Geometry check sheet. Reference: the model listing, model coordinates, mm. Face numbers are marked on the shaded views. A direction names the side the tool comes from. Round coordinates to 2 decimals unless told otherwise and drop trailing zeros. Write each loop counter-clockwise with the first axis right and the second up, starting at its lowest first coordinate (ties: lowest second). Pieces come first, ordered by that corner, then holes. Notation, with made-up numbers: M 56,64.25 L 93,64.25 A24 ccw 93,94.25 Z; hole C 61,43.25 d6. An arc over 180 degrees is marked long. Answer in a Markdown table with one row per item. Add a question column.
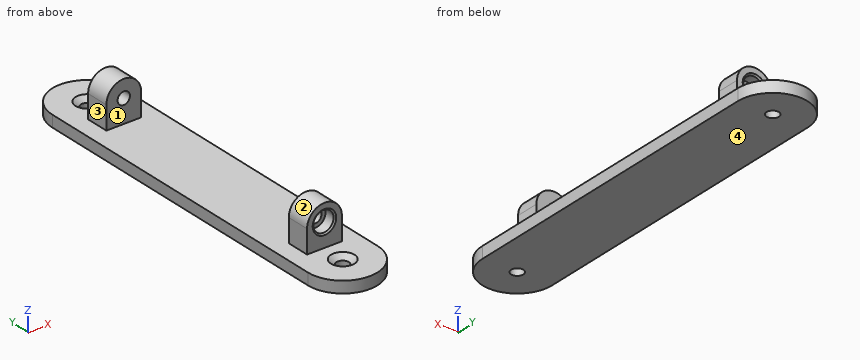
from build123d import *

# Parameters (mm, degrees)
BOSS_EXTRUDE1_DEPTH                                 = 6.35
CSK_FOR_1_4_FLAT_HEAD_MACHINE_SCREW_100_D           = 6.7564
CSK_FOR_1_4_FLAT_HEAD_MACHINE_SCREW_100_CSINK_D     = 12.8778
CSK_FOR_1_4_FLAT_HEAD_MACHINE_SCREW_100_CSINK_ANGLE = 100
SKETCH4_W                                           = 19.05
SKETCH4_H                                           = 12.7
BOSS_EXTRUDE2_DEPTH                                 = 12.7
BOSS_EXTRUDE4_DEPTH                                 = 12.7


with BuildPart() as part:
    # Sketch1 → Boss-Extrude1 (new body)
    with BuildSketch(Plane.XY):
        with BuildLine():
            Line((0, 0), (38.1, 0))
            Line((38.1, 0), (38.1, 88.9))
            ThreePointArc((38.1, 88.9), (19.05, 107.95), (0, 88.9))
            Line((0, 88.9), (0, 0))
        make_face()
    boss_extrude1 = extrude(amount=BOSS_EXTRUDE1_DEPTH)

    # CSK for 1/4 Flat Head Machine Screw (100)1 (through all)
    with Locations(Plane.XY.offset(6.35)):
        with Locations((19.05, 88.9)):
            csk_for_1_4_flat_head_machine_screw_100 = CounterSinkHole(CSK_FOR_1_4_FLAT_HEAD_MACHINE_SCREW_100_D / 2, CSK_FOR_1_4_FLAT_HEAD_MACHINE_SCREW_100_CSINK_D / 2, counter_sink_angle=CSK_FOR_1_4_FLAT_HEAD_MACHINE_SCREW_100_CSINK_ANGLE)

    # Sketch4 → Boss-Extrude2 (add)
    with BuildSketch(Plane.XY.offset(6.35)):
        with Locations((19.05, 69.85)):
            Rectangle(SKETCH4_W, SKETCH4_H)
    boss_extrude2 = extrude(amount=BOSS_EXTRUDE2_DEPTH)

    # Sketch12 → Boss-Extrude4 (add)
    with BuildSketch(Plane(origin=(0, 76.2, 0), x_dir=(1, 0, 0), z_dir=(0, 1, 0))):
        with BuildLine():
            Line((9.525, -19.05), (28.575, -19.05))
            ThreePointArc((28.575, -19.05), (19.05, -28.575), (9.525, -19.05))
        make_face()
    boss_extrude4 = extrude(amount=-BOSS_EXTRUDE4_DEPTH)

    # Sketch14 → CBORE for 1/4 Socket Head Cap Screw1 (revolve, cut)
    with BuildSketch(Plane(origin=(19.05, 76.2, 19.05), x_dir=(0, 0, 1), z_dir=(1, 0, 0))):
        Polygon((0, 0), (0, 141.728827343), (3.3782, 139.699), (3.3782, 6.35), (5.55625, 6.35), (5.55625, 0.740631289), (6.4389, 0), align=None)
    cbore_for_1_4_socket_head_cap_screw1 = revolve(axis=Axis((19.05, 82.55, 19.05), (0, -1, 0)), mode=Mode.SUBTRACT)

    # Mirror3: Boss-Extrude1, CSK for 1/4 Flat Head Machine Screw (100)1, Boss-Extrude2, Boss-Extrude4, CBORE for 1/4 Socket Head Cap Screw1 across plane
    add(boss_extrude1.mirror(Plane(origin=(0, 0, 6.35), x_dir=(0, 0, 1), z_dir=(0, 1, 0))))
    add(csk_for_1_4_flat_head_machine_screw_100.mirror(Plane(origin=(0, 0, 6.35), x_dir=(0, 0, 1), z_dir=(0, 1, 0))), mode=Mode.SUBTRACT)
    add(boss_extrude2.mirror(Plane(origin=(0, 0, 6.35), x_dir=(0, 0, 1), z_dir=(0, 1, 0))))
    add(boss_extrude4.mirror(Plane(origin=(0, 0, 6.35), x_dir=(0, 0, 1), z_dir=(0, 1, 0))))
    add(cbore_for_1_4_socket_head_cap_screw1.mirror(Plane(origin=(0, 0, 6.35), x_dir=(0, 0, 1), z_dir=(0, 1, 0))), mode=Mode.SUBTRACT)


solid = part.part
Item 1: Section check A-A, the plane z = 9.5. Record the boundary of the cut face in (x, y) (3 decimals).
Item 2: Access from +Z, -Z, +X, -X, +Y, -Y to the whole of each face (thin tool, end or side, straight path). Record for the marked faces 3 and 4.
Item 3: Section check C-C, the plane y = 23.5. Record the boundary of the cut face in (x, z), and give its area (3 significant figures).
Item 4: Gauge pin test, flat ends, axial feed: pin 1 Ø5.5 at (x, z) = (17.5, 20.5) entering from -Y; pin 2 Ø10 at (x, z) = (14, 4.5) entering from +Y; pin 3 Ø9.5 at (x, z) = (19.5, 14) entering from +Y. Record the tip position at first contact, or that the pin passes through.
Item 5: Section check D-D, the plane x = 31.5. Record the boundary of the cut face in (y, z).
Item 6: Section check B-B, the plane x = 19.05. Give the number of separate pieces and of enclosed holes in the cut face, and give its area (3 significant figures).
Item 7: Mould release check, pull along Y, two halves, no side actions. Record for the marked faces 1 and 2: +Y half, -Y half, draft (parallel to the pull), parting line (faces both ways), or undercut.
Item 8: Scan lines: probe 1 along Y at (x, z) = (19.05, 1.4); probe 2 along Y at (x, z) = (12, 16.5); probe 3 along Z at (x, y) = (19.05, -66.75) (3 decimals). Record each from-to range of solid material in increasing order. Write a range as from..to.
Result sheet:
| question | item | result |
|---|---|---|
| 1 | outline | M 9.525,-76.2 L 28.575,-76.2 L 28.575,-63.5 L 9.525,-63.5 Z; M 9.525,63.5 L 28.575,63.5 L 28.575,76.2 L 9.525,76.2 Z |
| 2 | face 3 | +Z, -X, +Y, -Y |
| 2 | face 4 | -Z, +X, -X, +Y, -Y |
| 3 | outline | M 0,0 L 38.1,0 L 38.1,6.35 L 0,6.35 Z |
| 3 | area | 242 mm^2 |
| 4 | pin 1 | stops at y = -69.85 |
| 4 | pin 2 | stops at y = 107.95 |
| 4 | pin 3 | stops at y = 76.2 |
| 5 | outline | M -103.32,0 L 103.32,0 L 103.32,6.35 L -103.32,6.35 Z |
| 6 | separate pieces | 5 |
| 6 | enclosed holes | 0 |
| 6 | area | 1,610 mm^2 |
| 7 | face 1 | undercut |
| 7 | face 2 | draft |
| 8 | probe 1 | y = -107.95..-92.28, -85.52..85.52, 92.28..107.95 |
| 8 | probe 2 | y = -76.2..-63.5, 63.5..76.2 |
| 8 | probe 3 | z = 0..15.672, 22.428..28.575 |
